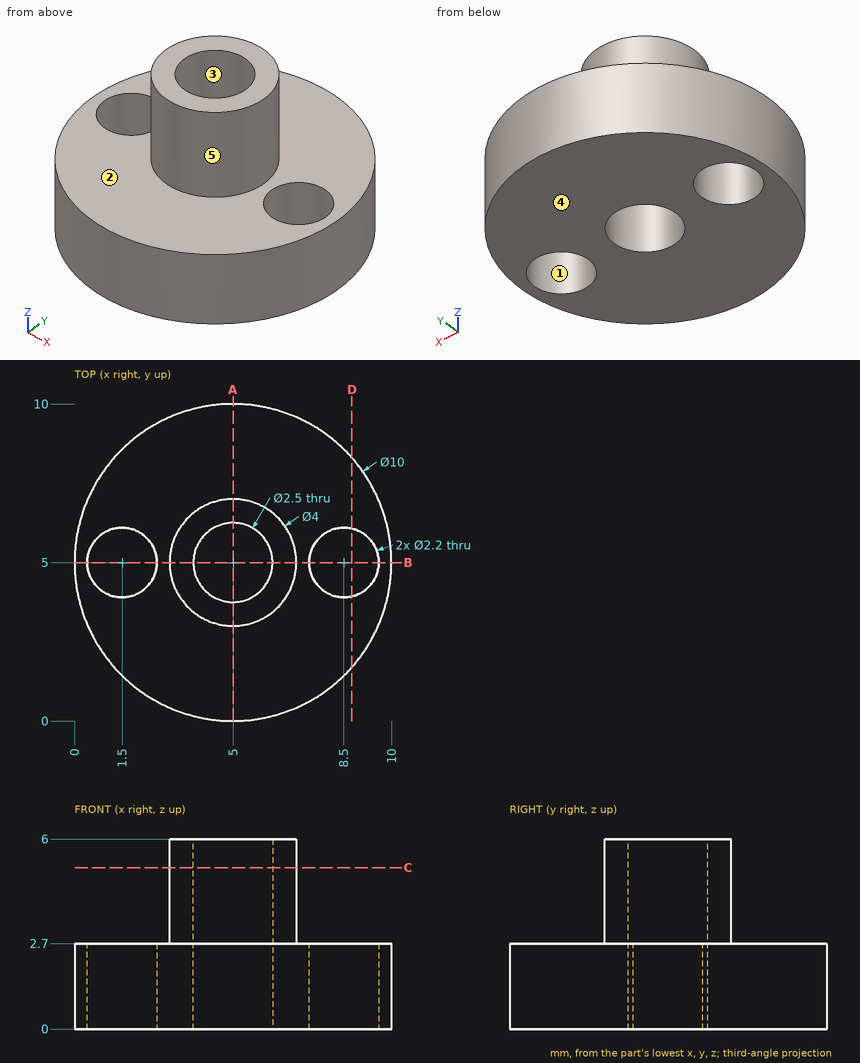
Input: dimensioned drawing with shaded views. Units: mm. Origin: part minimum x, y, z. A direction names the side the tool comes from. Coordinates: 2 decimals unless noted, no trailing zeros. Order: outer loops, then holes, each group sorted by start corner. A loop starts at its lowest first (then second) coordinate and runs counter-clockwise, first axis right, second up. Notation, with made-up numbers: (66, -18.5) - (92, -18.5) arc R14 ccw to (92, -9.5) - close; hole circle Ø2 at (66.25, 47). An arc over 180 degrees is marked (long way). One line per item, written item: value.
1) Ray query, line 1 (Z direction, x = 3.5, y = 9.5); line 2 (Y direction, x = 8.75, z = 0.4); line 3 (Y direction, x = 1.5, z = 1.3). Return the intervals inside material, ascending. Write a range as [from, to].
Computed values:
line 1: z = [0, 2.7]
line 2: y = [1.69, 3.93], [6.07, 8.31]
line 3: y = [1.43, 3.9], [6.1, 8.57]
2) Cut plane A-A on x = 5. Output: boundary loops of the cut face in (y, z).
Computed values:
outline: (0, 0) - (3.75, 0) - (3.75, 6) - (3, 6) - (3, 2.7) - (0, 2.7) - close; (6.25, 0) - (10, 0) - (10, 2.7) - (7, 2.7) - (7, 6) - (6.25, 6) - close
3) Mould query, pull axis X, two halves, no side actions, for the marked faces 3, 4 and 5. Classes: released by +X, released by -X, zero draft, split by the parting line, or undercut.
Computed values:
face 3: undercut
face 4: zero draft
face 5: split by the parting line
4) Cut plane D-D on x = 8.75. Output: boundary loops of the cut face in (y, z).
Computed values:
outline: (1.69, 0) - (3.93, 0) - (3.93, 2.7) - (1.69, 2.7) - close; (6.07, 0) - (8.31, 0) - (8.31, 2.7) - (6.07, 2.7) - close
5) Reachability of the marked faces 1 and 2 from +Z, -Z, +X, -X, +Y, -Y: full face, straight path, thin tool, end or side. Return the list, or none.
Computed values:
face 1: +Z, -Z
face 2: +Z
6) Cut plane C-C on z = 5.1. Output: boundary loops of the cut face in (x, y), plus the area to 3 significant figures.
Computed values:
outline: circle Ø4 at (5, 5); hole circle Ø2.5 at (5, 5)
area: 7.66 mm^2
7) Contact query for flat-ended pins moving along their axis: pin 1 (1.5 mm diameter, centred on x = 5, y = 5, fed in from +Z); pin 2 (1 mm diameter, centred on y = 8, z = 1.5, fed in from +X). Output: stop coordinate, or through.
Computed values:
pin 1: passes through
pin 2: stops at x = 9.33
8) Cut plane B-B on y = 5. Output: boundary loops of the cut face in (x, z), plus the area to 3 significant figures.
Computed values:
outline: (0, 0) - (0.4, 0) - (0.4, 2.7) - (0, 2.7) - close; (2.6, 0) - (3.75, 0) - (3.75, 6) - (3, 6) - (3, 2.7) - (2.6, 2.7) - close; (6.25, 0) - (7.4, 0) - (7.4, 2.7) - (7, 2.7) - (7, 6) - (6.25, 6) - close; (9.6, 0) - (10, 0) - (10, 2.7) - (9.6, 2.7) - close
area: 13.3 mm^2
